Model file for the job. Use its own axes, mm. Face numbers are marked on the shaded views. A direction names the side the tool comes from. Give positions to 0.01 mm unless a question says otherwise; leave off trailing zeros. Loops run counter-clockwise (first coordinate to the right, second up) from the corner with the lowest first, then second, coordinate; pieces in that order, holes last. Notation, with made-up numbers: M 72.5,-39.5 L 87.5,-39.5 A30 cw 87.5,-11.5 Z; hole C 25.25,34 d9. An arc over 180 degrees is marked long. Use CSV: the item, a comma, the result in double quotes. Start each with the question number.
(1) Slice it at A-A on x = 37. List the corners of the cut face in (y, z), and give its area (3 significant figures).
(2) Slice it at B-B on z = 10.5. List the corners of the cut face in (x, y).
(3) Wall check: line 1 along X through (y, z) = (-13, 18.5); line 2 along X through (y, z) = (-88, 26); line 3 along Y through (x, z) = (83, 101.5). Give the ranges that are in metal, low to high. Write a range as from..to.
(4) Two-plate mould, pull along X, no slides. Class the marked faces 1, 2 and 3: pulls with the +X half, pulls with the -X half, needs draft (parallel to the pull), parting line crosses it, or undercut.
(5) Slice it at C-C on y = -20. List the corners of the cut face in (x, z).
(6) Flat gauge pins, fed straight in: P1, Ø3, axis at y = -90, z = -57.5, coming from the -X side; P2, Ø12, axis at x = 211.5, z = 45.5, coming from the -Y side; P3, Ø1, axis at y = -167.5, z = 49, coming from the -X side. Where does each tip first touch, or does it go through?
(7) Tool access for the marked faces 4 and 5: list every direction of +Z, -Z, +X, -X, +Y, -Y with a clear straight run to the whole face (end or side of a thin tool).
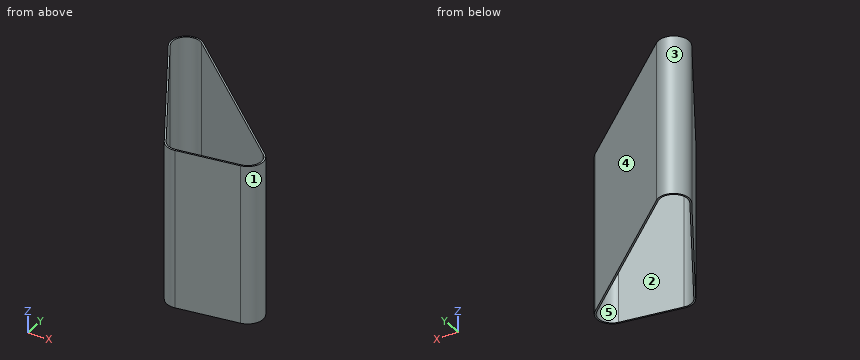
```python
from build123d import *

# Parameters (mm, degrees)
ESQUISSE3_W = 290
ESQUISSE3_H = 3


with BuildPart() as part:
    # Balayage1: sweep along a path in Esquisse2
    with BuildLine(Plane.XY) as balayage1_path:
        Line((-21.650635095, -12.5), (116.913429511, -252.5))
        ThreePointArc((116.913429511, -252.5), (127.558761221, -262.447344997), (141.941894724, -264.770754201))
        Line((141.941894724, -264.770754201), (251.941894724, -249.770754201))
        ThreePointArc((251.941894724, -249.770754201), (272.446913518, -232.389825968), (265.341354263, -206.465638621))
        Line((265.341354263, -206.465638621), (16.777289658, 18.534361379))
        ThreePointArc((16.777289658, 18.534361379), (-15.707331743, 19.449414631), (-21.650635095, -12.5))
    # Esquisse3 → Balayage1 (sweep)
    with BuildSketch(Plane(origin=(0, 0, 0), x_dir=(0, 0, -1), z_dir=(1, 0, 0))):
        with Locations((0, 26.5)):
            Rectangle(ESQUISSE3_W, ESQUISSE3_H)
    sweep(path=balayage1_path.line)


solid = part.part
```
Reply:
1,outline,"M -120.09,-145 L -114.09,-145 L -114.09,145 L -120.09,145 Z; M 0.23,-145 L 4.28,-145 L 4.28,145 L 0.23,145 Z"
1,area,"2,910 mm^2"
2,outline,"M -24.25,-14 L 114.32,-254 A28 ccw 142.35,-267.74 L 252.35,-252.74 A28 ccw 267.35,-204.24 L 18.79,20.76 A28 ccw Z; hole M -21.65,-12.5 L 116.91,-252.5 A25 ccw 141.94,-264.77 L 251.94,-249.77 A25 ccw 265.34,-206.47 L 16.78,18.53 A25 ccw Z"
3,line 1,"x = -24.8..-21.36, 51.61..56.08"
3,line 2,"x = 18.48..21.94, 134.47..138.94"
3,line 3,"y = -199.76..-193.76, -41.41..-37.36"
4,face 1,"pulls with the +X half"
4,face 2,"undercut"
4,face 3,"parting line crosses it"
5,outline,"M -20.78,-145 L -17.32,-145 L -17.32,145 L -20.78,145 Z; M 59.35,-145 L 63.82,-145 L 63.82,145 L 59.35,145 Z"
6,P1,"stops at x = 18.76"
6,P2,"stops at y = -259.13"
6,P3,"stops at x = 64.09"
7,face 4,"+Z, -Z, +X, +Y"
7,face 5,"+Z, -Z"
